The listing builds one solid part. Answer for the finished solid, in the listing's coordinates (mm). Face numbers are marked on the shaded views. Coordinates: 2 decimals unless noted, no trailing zeros. Loops run counter-clockwise (first coordinate to the right, second up) from the corner with the lowest first, then second, coordinate; pieces in that order, holes last. Notation, with made-up numbers: M 38,0 L 51,0 A24 cw 51,28 Z; hole C 22.5,52 d10. An arc over 180 degrees is marked long. Answer as a JSON object with one key per item and string values. Group by question number.
1. Given pin 1 (2 mm diameter, centred on x = 8.5, y = 79.5, fed in from +Z); pin 2 (0.8 mm diameter, centred on x = 33.5, y = 20.5, fed in from +Z); pin 3 (14 mm diameter, centred on x = 18, y = 59, fed in from +Z), each flat-ended and moving along its own axis, determine where each tip first touches the part or whether it passes through.
2. A cutting plane is placed at B-B on y = 63. Give the vertices of the cut face in (x, z).
3. A cutting plane is placed at C-C on x = 9. Give the vertices of the cut face in (y, z), and give its area (3 significant figures).
4. Determine the mould class of the marked faces 1 and 2 for opening direction X: released by +X, released by -X, zero draft, split by the parting line, or undercut.
5. Straight lines are drawn through the part: L1, parallel to Y at x = 21, z = 2; L2, parallel to X at y = 32, z = 2.5; L3, parallel to Z at x = 32, y = 65. For each, find the intervals that lie inside material, in ascending order.
6. A cutting plane is placed at A-A on z = 1. Give the vertices of the cut face in (x, y), and give its area (3 significant figures).
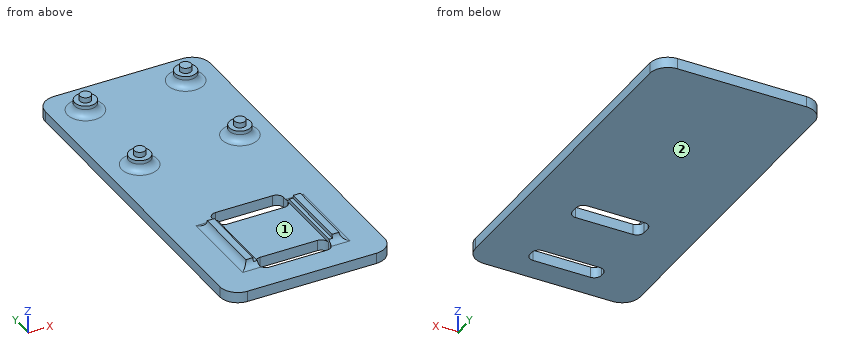
from build123d import *

# Parameters (mm, degrees)
SKETCH_1_W          = 46
SKETCH_1_H          = 100
EXTRUDE_1_DEPTH     = 3
SKETCH_2_R          = 3
EXTRUDE_2_DEPTH     = 3
SKETCH_3_R          = 1.55
EXTRUDE_3_DEPTH     = 1.5
FILLET_1_R          = 2
FILLET_2_R          = 5
SKETCH_4_W          = 2
SKETCH_4_H          = 20
SKETCH_4_W_2        = 1
EXTRUDE_4_DEPTH     = 2
SKETCH_5_W          = 22.1
SKETCH_5_H          = 30
CUT_EXTRUDE_1_DEPTH = 1
FILLET_3_R          = 2
SKETCH_6_W          = 20
SKETCH_6_H          = 6
SKETCH_6_H_2        = 5
CUT_EXTRUDE_2_DEPTH = 10
FILLET_4_R          = 2


with BuildPart() as part:
    # ｽｹｯﾁ1 → ﾎﾞｽ - 押し出し1 (new body)
    with BuildSketch(Plane.XY):
        with Locations((23, 50)):
            Rectangle(SKETCH_1_W, SKETCH_1_H)
    extrude(amount=EXTRUDE_1_DEPTH)

    # ｽｹｯﾁ2 → ﾎﾞｽ - 押し出し2 (add)
    with BuildSketch(Plane.XY.offset(3)):
        with Locations(Location((9, 91, 0), (0, 0, 180))):
            Circle(SKETCH_2_R)
        with Locations(Location((37, 91, 0), (0, 0, 180))):
            Circle(SKETCH_2_R)
        with Locations(Location((9, 63, 0), (0, 0, 180))):
            Circle(SKETCH_2_R)
        with Locations(Location((37, 63, 0), (0, 0, 180))):
            Circle(SKETCH_2_R)
    extrude(amount=EXTRUDE_2_DEPTH)

    # ｽｹｯﾁ3 → ﾎﾞｽ - 押し出し3 (add)
    with BuildSketch(Plane.XY.offset(6)):
        with Locations((9, 91)):
            Circle(SKETCH_3_R)
        with Locations((37, 91)):
            Circle(SKETCH_3_R)
        with Locations((9, 63)):
            Circle(SKETCH_3_R)
        with Locations((37, 63)):
            Circle(SKETCH_3_R)
    extrude(amount=EXTRUDE_3_DEPTH)

    # ﾌｨﾚｯﾄ1
    fillet_1_edges = [part.edges().sort_by_distance(p)[0] for p in [
        (12, 91, 3),
        (40, 91, 3),
        (12, 63, 3),
        (40, 63, 3),
    ]]
    fillet(fillet_1_edges, radius=FILLET_1_R)

    # ﾌｨﾚｯﾄ2
    fillet_2_edges = [part.edges().sort_by_distance(p)[0] for p in [
        (0, 100, 1.5),
        (46, 100, 1.5),
        (46, 0, 1.5),
        (0, 0, 1.5),
    ]]
    fillet(fillet_2_edges, radius=FILLET_2_R)

    # ｽｹｯﾁ4 → ﾎﾞｽ - 押し出し4 (add)
    with BuildSketch(Plane.XY.offset(3)):
        with Locations((11, 20)):
            Rectangle(SKETCH_4_W, SKETCH_4_H)
        with Locations((12.5, 20)):
            Rectangle(SKETCH_4_W_2, SKETCH_4_H)
        with Locations((33.5, 20)):
            Rectangle(SKETCH_4_W_2, SKETCH_4_H)
        with Locations((35, 20)):
            Rectangle(SKETCH_4_W, SKETCH_4_H)
    extrude(amount=EXTRUDE_4_DEPTH)

    # ｽｹｯﾁ5 → ｶｯﾄ - 押し出し1 (cut)
    with BuildSketch(Plane.XY.offset(5)):
        with Locations((23, 20)):
            Rectangle(SKETCH_5_W, SKETCH_5_H)
    extrude(amount=-CUT_EXTRUDE_1_DEPTH, mode=Mode.SUBTRACT)

    # ﾌｨﾚｯﾄ3
    fillet_3_edges = [part.edges().sort_by_distance(p)[0] for p in [
        (11.5, 30, 3),
    ]]
    fillet(fillet_3_edges, radius=FILLET_3_R - 0.0001)  # a hair under: the kernel refuses the full size
    fillet_3_2_edges = [part.edges().sort_by_distance(p)[0] for p in [
        (10, 20, 3),
    ]]
    fillet(fillet_3_2_edges, radius=FILLET_3_R - 0.0001)  # a hair under: the kernel refuses the full size
    fillet_3_3_edges = [part.edges().sort_by_distance(p)[0] for p in [
        (11.5, 10, 3),
    ]]
    fillet(fillet_3_3_edges, radius=FILLET_3_R - 0.0001)  # a hair under: the kernel refuses the full size
    fillet_3_4_edges = [part.edges().sort_by_distance(p)[0] for p in [
        (34.5, 30, 3),
    ]]
    fillet(fillet_3_4_edges, radius=FILLET_3_R - 0.0004)  # a hair under: the kernel refuses the full size
    fillet_3_5_edges = [part.edges().sort_by_distance(p)[0] for p in [
        (34.5, 10, 3),
    ]]
    fillet(fillet_3_5_edges, radius=FILLET_3_R - 0.0004)  # a hair under: the kernel refuses the full size
    fillet_3_6_edges = [part.edges().sort_by_distance(p)[0] for p in [
        (36, 20, 3),
    ]]
    fillet(fillet_3_6_edges, radius=FILLET_3_R - 0.0004)  # a hair under: the kernel refuses the full size

    # ｽｹｯﾁ6 → ｶｯﾄ - 押し出し2 (cut)
    with BuildSketch(Plane.XY.offset(3)):
        with Locations((23, 32)):
            Rectangle(SKETCH_6_W, SKETCH_6_H)
        with Locations((23, 9.5)):
            Rectangle(SKETCH_6_W, SKETCH_6_H_2)
    extrude(amount=-CUT_EXTRUDE_2_DEPTH, mode=Mode.SUBTRACT)

    # ﾌｨﾚｯﾄ4
    fillet_4_edges = [part.edges().sort_by_distance(p)[0] for p in [
        (13, 29, 1.5),
        (13, 35, 1.5),
        (33, 35, 1.5),
        (33, 29, 1.5),
        (13, 7, 1.5),
        (13, 12, 1.5),
        (33, 12, 1.5),
        (33, 7, 1.5),
    ]]
    fillet(fillet_4_edges, radius=FILLET_4_R)


solid = part.part
From the geometry:
{
 "1": {"pin 1": "stops at z = 3", "pin 2": "stops at z = 4", "pin 3": "stops at z = 6"},
 "2": {"outline": "M 0,0 L 46,0 L 46,3 L 42,3 A2 cw 40,5 L 40,6 L 38.55,6 L 38.55,7.5 L 35.45,7.5 L 35.45,6 L 34,6 L 34,5 A2 cw 32,3 L 14,3 A2 cw 12,5 L 12,6 L 10.55,6 L 10.55,7.5 L 7.45,7.5 L 7.45,6 L 6,6 L 6,5 A2 cw 4,3 L 0,3 Z"},
 "3": {"outline": "M 0,0 L 100,0 L 100,3 L 96,3 A2 cw 94,5 L 94,6 L 92.55,6 L 92.55,7.5 L 89.45,7.5 L 89.45,6 L 88,6 L 88,5 A2 cw 86,3 L 68,3 A2 cw 66,5 L 66,6 L 64.55,6 L 64.55,7.5 L 61.45,7.5 L 61.45,6 L 60,6 L 60,5 A2 cw 58,3 L 32,3 A2 cw 31,3.27 L 9,3.27 A2 cw 8,3 L 0,3 Z", "area": "355 mm²"},
 "4": {"face 1": "undercut", "face 2": "zero draft"},
 "5": {"L1": "y = 0 to 7, 12 to 29, 35 to 100", "L2": "x = 0 to 13, 33 to 46", "L3": "z = 0 to 3"},
 "6": {"outline": "M 0,5 A5 ccw 5,0 L 41,0 A5 ccw 46,5 L 46,95 A5 ccw 41,100 L 5,100 A5 ccw 0,95 Z; hole M 13,9 A2 ccw 15,7 L 31,7 A2 ccw 33,9 L 33,10 A2 ccw 31,12 L 15,12 A2 ccw 13,10 Z; hole M 13,31 A2 ccw 15,29 L 31,29 A2 ccw 33,31 L 33,33 A2 ccw 31,35 L 15,35 A2 ccw 13,33 Z", "area": "4,370 mm²"}
}
